The model under review builds one solid part; all positions refer to its coordinate system, in mm. Face numbers are marked on the shaded views. A direction names the side the tool comes from. Coordinates: 2 decimals unless noted, no trailing zeros. Write each loop counter-clockwise with the first axis right and the second up, starting at its lowest first coordinate (ties: lowest second). Pieces come first, ordered by that corner, then holes. Notation, with made-up numbers: (12, -26.5) - (39, -26.5) arc R14 ccw to (39, -20.5) - close; hole circle Ø8 at (20, -8.75). An arc over 180 degrees is marked (long way). Return JSON: item names as keys, results as strings. Group by question number.
(1) We need section A-A on z = -5.75. State the section outline as (x, y) points, then the cut area to 3 significant figures.
(2) To check wall thickness, follow L1, parallel to Y at x = 62, z = -6.75; L2, parallel to Z at x = -110, y = 16.5; L3, parallel to Y at x = -99, z = -22.25. State the ranges of each line that lie inside material, in increasing order. Write a range as from..to.
(3) Tool access review of the marked faces 1 and 2: name each direction out of +Z, -Z, +X, -X, +Y, -Y from which nothing blocks a thin tool from reaching the whole face with its end or side.
(4) We need section B-B on y = -10. State the section outline as (x, z) points.
(5) We need section C-C on z = -24.75. State the section outline as (x, y) points.
(6) We need section D-D on x = 30. State the section outline as (y, z) points.
(7) For pin 1 Ø8 at (x, z) = (4, -17.5) entering from -Y; pin 2 Ø0.6 at (x, y) = (4.5, -21.5) entering from -Z; pin 3 Ø10 at (y, z) = (-24.5, -13.5) entering from -X; pin 4 Ø18 at (x, y) = (36.5, -4) entering from -Z, all flat-tipped, find the tip position at first contact; note any pin that passes through.
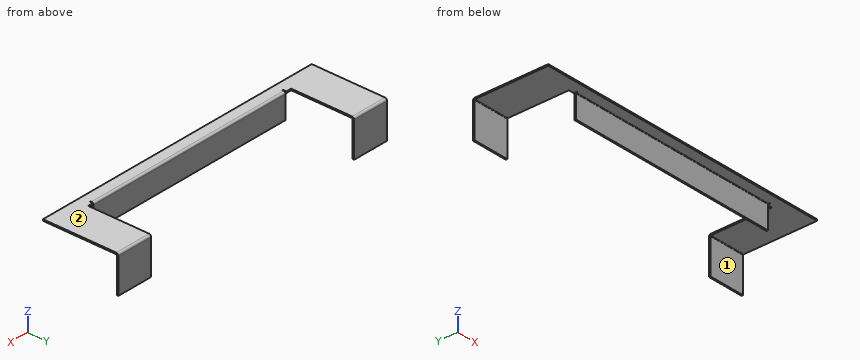
```python
from build123d import *

# Parameters (mm, degrees)
SKETCH_2_W                         = 245.6
SKETCH_2_H                         = 61.2
SM_BASE_FLANGE_1_DEPTH             = 1.2
SKETCH_8_W                         = 185.6
SKETCH_8_H                         = 51.2
CUT_EXTRUDE_1_DEPTH                = 10
SM_EDGE_FLANGE_1_STRIP_W           = 5.8
SM_EDGE_FLANGE_1_STRIP_H           = 1.2
SM_EDGE_FLANGE_1_STRIP_CUT_DEPTH   = 30
SM_EDGE_FLANGE_1_STRIP_2_W         = 5.8
SM_EDGE_FLANGE_1_STRIP_2_H         = 1.2
SM_EDGE_FLANGE_1_STRIP_CUT_2_DEPTH = 30
SM_EDGE_FLANGE_1_DEPTH             = 30
SM_EDGE_FLANGE_1_BEND_DEPTH        = 30
SM_START                           = -1.7
SM_EDGE_FLANGE_2_DEPTH             = 2.7
SM_START_2                         = -20
SM_EDGE_FLANGE_2_2_OUTLINE_W       = 175.6
SM_EDGE_FLANGE_2_2_OUTLINE_H       = 1.2
SM_EDGE_FLANGE_2_2_DEPTH           = 18.3
SM_START_3                         = -87.8
SM_EDGE_FLANGE_2_3_DEPTH           = 175.6
SM_EDGE_FLANGE_2_4_DEPTH           = 175.6


with BuildPart() as part:
    # 基体-法兰1: sheet metal written as solids
    # Sketch 2 → 基体-法兰1 (new body)
    with BuildSketch(Plane.XY):
        Rectangle(SKETCH_2_W, SKETCH_2_H)
    extrude(amount=-SM_BASE_FLANGE_1_DEPTH)

    # 草图8 → 切除-拉伸1 (cut)
    with BuildSketch(Plane.XY):
        with Locations((0, 5)):
            Rectangle(SKETCH_8_W, SKETCH_8_H)
    extrude(amount=-CUT_EXTRUDE_1_DEPTH, mode=Mode.SUBTRACT)

    # 边线-法兰1: sheet metal written as solids
    # 边线-法兰1 strip (on a plane across the edge) → 边线-法兰1 strip cut (cut)
    with BuildSketch(Plane(origin=(92.8, 30.6, -1.2), x_dir=(0, -1, 0), z_dir=(1, 0, 0))):
        with Locations((-1.2, -0.6)):
            Rectangle(SM_EDGE_FLANGE_1_STRIP_W, SM_EDGE_FLANGE_1_STRIP_H)
    extrude(amount=SM_EDGE_FLANGE_1_STRIP_CUT_DEPTH, mode=Mode.SUBTRACT)

    # 边线-法兰1 strip 2 (on a plane across the edge) → 边线-法兰1 strip cut 2 (cut)
    with BuildSketch(Plane(origin=(-122.8, 30.6, -1.2), x_dir=(0, -1, 0), z_dir=(1, 0, 0))):
        with Locations((-1.2, -0.6)):
            Rectangle(SM_EDGE_FLANGE_1_STRIP_2_W, SM_EDGE_FLANGE_1_STRIP_2_H)
    extrude(amount=SM_EDGE_FLANGE_1_STRIP_CUT_2_DEPTH, mode=Mode.SUBTRACT)

    # 边线-法兰1 section (on a plane across the edge) → 边线-法兰1 (add)
    with BuildSketch(Plane(origin=(92.8, 30.6, -1.2), x_dir=(0, -1, 0), z_dir=(1, 0, 0))):
        with BuildLine():
            Line((0, 0.5), (0, 28.8))
            Line((0, 28.8), (1.2, 28.8))
            Line((1.2, 28.8), (1.2, 0.5))
            ThreePointArc((1.2, 0.5), (1.346446609, 0.146446609), (1.7, 0))
            Line((1.7, 0), (1.7, -1.2))
            ThreePointArc((1.7, -1.2), (0.497918472, -0.702081528), (0, 0.5))
        make_face()
    extrude(amount=SM_EDGE_FLANGE_1_DEPTH)

    # 边线-法兰1 section 2 (on a plane across the edge) → 边线-法兰1 bend (add)
    with BuildSketch(Plane(origin=(-122.8, 30.6, -1.2), x_dir=(0, -1, 0), z_dir=(1, 0, 0))):
        with BuildLine():
            Line((0, 0.5), (0, 28.8))
            Line((0, 28.8), (1.2, 28.8))
            Line((1.2, 28.8), (1.2, 0.5))
            ThreePointArc((1.2, 0.5), (1.346446609, 0.146446609), (1.7, 0))
            Line((1.7, 0), (1.7, -1.2))
            ThreePointArc((1.7, -1.2), (0.497918472, -0.702081528), (0, 0.5))
        make_face()
    extrude(amount=SM_EDGE_FLANGE_1_BEND_DEPTH)

    # 边线-法兰2: read off the stored shape, not the designer's step
    # 边线-法兰2 outline → 边线-法兰2 (cut)
    with BuildSketch(Plane.XY.offset(SM_START)):
        with BuildLine():
            Line((-87.8, -22.9), (-87.8, -20.6))
            Line((-87.8, -20.6), (-88.4, -20.6))
            Line((-88.4, -20.6), (-88.4, -22.9))
            ThreePointArc((-88.4, -22.9), (-88.1, -23.2), (-87.8, -22.9))
        make_face()
        with BuildLine():
            Line((88.4, -20.6), (87.8, -20.6))
            Line((87.8, -20.6), (87.8, -22.9))
            ThreePointArc((87.8, -22.9), (88.1, -23.2), (88.4, -22.9))
            Line((88.4, -22.9), (88.4, -20.6))
        make_face()
    extrude(amount=SM_EDGE_FLANGE_2_DEPTH, mode=Mode.SUBTRACT)

    # Sm Edge Flange 2 3 outline → Sm Edge Flange 2 3 (cut)
    with BuildSketch(Plane.YZ.offset(SM_START_3)):
        with BuildLine():
            ThreePointArc((-22.3, 0), (-21.290049506, -0.332520567), (-20.675192319, -1.2))
            Line((-20.675192319, -1.2), (-20.6, -1.2))
            Line((-20.6, -1.2), (-20.6, 0))
            Line((-20.6, 0), (-22.3, 0))
        make_face()
    extrude(amount=SM_EDGE_FLANGE_2_3_DEPTH, mode=Mode.SUBTRACT)



with BuildPart() as body_2:
    # Sm Edge Flange 2 2 outline → Sm Edge Flange 2 2 (new body)
    with BuildSketch(Plane.XY.offset(SM_START_2)):
        with Locations((0, -21.2)):
            Rectangle(SM_EDGE_FLANGE_2_2_OUTLINE_W, SM_EDGE_FLANGE_2_2_OUTLINE_H)
    extrude(amount=SM_EDGE_FLANGE_2_2_DEPTH)


with BuildPart() as part_1:
    add(part.part)

    add(body_2.part)  # Sm Edge Flange 2 4 merges body 2
    # Sm Edge Flange 2 4 outline → Sm Edge Flange 2 4 (add)
    with BuildSketch(Plane.YZ.offset(SM_START_3)):
        with BuildLine():
            Line((-21.8, -1.7), (-20.6, -1.7))
            ThreePointArc((-20.6, -1.7), (-20.618903177, -1.447188863), (-20.675192319, -1.2))
            Line((-20.675192319, -1.2), (-22.3, -1.2))
            ThreePointArc((-22.3, -1.2), (-21.946446609, -1.346446609), (-21.8, -1.7))
        make_face()
    extrude(amount=SM_EDGE_FLANGE_2_4_DEPTH)


solid = part_1.part
```
Ans:
{
 "1": {"outline": "(-122.8, 29.4) - (-92.8, 29.4) - (-92.8, 30.6) - (-122.8, 30.6) - close; (-87.8, -21.8) - (87.8, -21.8) - (87.8, -20.6) - (-87.8, -20.6) - close; (92.8, 29.4) - (122.8, 29.4) - (122.8, 30.6) - (92.8, 30.6) - close", "area": "283 mm²"},
 "2": {"L1": "-21.8..-20.6", "L2": "-1.2..0", "L3": "29.4..30.6"},
 "3": {"face 1": "-Z, +X, -X, -Y", "face 2": "+Z, +X, -X, +Y, -Y"},
 "4": {"outline": "(-122.8, -1.2) - (-92.8, -1.2) - (-92.8, 0) - (-122.8, 0) - close; (92.8, -1.2) - (122.8, -1.2) - (122.8, 0) - (92.8, 0) - close"},
 "5": {"outline": "(-122.8, 29.4) - (-92.8, 29.4) - (-92.8, 30.6) - (-122.8, 30.6) - close; (92.8, 29.4) - (122.8, 29.4) - (122.8, 30.6) - (92.8, 30.6) - close"},
 "6": {"outline": "(-30.6, -1.2) - (-22.3, -1.2) arc R0.5 cw to (-21.8, -1.7) - (-21.8, -20) - (-20.6, -20) - (-20.6, -1.7) arc R1.7 ccw to (-22.3, 0) - (-30.6, 0) - close"},
 "7": {"pin 1": "y = -21.8", "pin 2": "z = -20", "pin 3": "x = -87.8", "pin 4": "through"}
}
